Geometry check sheet. Reference: the model listing, model coordinates, mm. A direction names the side the tool comes from. Give positions to 0.01 mm unless a question says otherwise; leave off trailing zeros. Write each loop counter-clockwise with the first axis right and the second up, starting at its lowest first coordinate (ties: lowest second). Pieces come first, ordered by that corner, then holes.
(1) Cross-section at D-D (z = -24.5). Record the boundary of the cut face in (x, y), and give its area (3 significant figures).
(2) Tool access check on faces 1 (the cylindrical face through (123.767, 0.021, -65.778)), 2 (the cylindrical face through (180.594, 0.021, -25.778)). Record the directions out of +Z, -Z, +X, -X, +Y, -Y that give a thin tool (end or side, any length) a straight path to the whole face; none if there is none.
(3) Cross-section at B-B (x = -94.5). Record the boundary of the cut face in (y, z), and give its area (3 significant figures).
(4) Depth check by flat-ended pin: P1, Ø1.5, axis at y = 0, z = -4.5, coming from the +X side; P2, Ø0.9, axis at y = -0.5, z = -73, coming from the +X side; P3, Ø2.5, axis at x = -101.25, z = -43.75, coming from the -Y side; P4, Ø1.5, axis at y = 0, z = -9.5, coming from the -X side. Enter the tip coordinate at first touch or a pass-through.
(5) Cross-section at A-A (y = 0.95). Count the separate pieces of the cut face and the enclosed holes in it, and give its area (3 significant figures).
(6) Thickness scan on line 1 along X through (y, z) = (0.2, -79); line 2 along X through (y, z) = (-0.5, -65.5); line 3 along Z through (x, y) = (113.5, -0.1). Record the ranges inside material, lowest first.
(7) Mould release check, pull along X, two halves, no side actions. Record for faces 3 (the flat face through (-3, 1.5, -71)), 4 (the cylindrical face through (59.49, 0.02, 10.9)), 5 (the cylindrical face through (-121.62, 0.02, -63.68)), 6 (the cylindrical face through (121.62, 0.02, -63.68)): +X half, -X half, draft (parallel to the pull), parting line (faces both ways), or undercut.
```python
from build123d import *

# Parameters (mm, degrees)
BOSS_EXTRUDE1_DEPTH      = 1.5
BOSS_EXTRUDE1_DEPTH_BACK = 1.5
SKETCH1_W                = 125
SKETCH1_H                = 27.5
FILLET1_R                = 10
FILLET2_R                = 10
BOSS_EXTRUDE2_DEPTH      = 1.5
BOSS_EXTRUDE2_DEPTH_BACK = 1.5
SKETCH3_W                = 384
SKETCH3_H                = 110
FILLET3_R                = 40
FILLET4_R                = 40
CUT_EXTRUDE1_DEPTH       = 229.444878472
FILLET5_R                = 40
FILLET5_OF_MIRROR1_R     = 40
SKETCH5_R                = 1.5
CUT_EXTRUDE2_DEPTH       = 229.444878611
SKETCH8_W                = 3
SKETCH8_H                = 3
CUT_REVOLVE1_ANGLE       = 90


with BuildPart() as part:
    # Sketch1 → Boss-Extrude1 (new, two sides: drawn at the far end of the back side and taken through both)
    with BuildSketch(Plane(origin=(0, 0, 0), x_dir=(1, 0, 0), z_dir=(0, 1, 0)).offset(-BOSS_EXTRUDE1_DEPTH_BACK)):
        Rectangle(SKETCH1_W, SKETCH1_H)
    extrude(amount=BOSS_EXTRUDE1_DEPTH + BOSS_EXTRUDE1_DEPTH_BACK)

    # Fillet1
    fillet1_edges = [part.edges().sort_by_distance(p)[0] for p in [
        (-62.5, 0, 13.75),
    ]]
    fillet(fillet1_edges, radius=FILLET1_R)

    # Fillet2
    fillet2_edges = [part.edges().sort_by_distance(p)[0] for p in [
        (62.5, 0, 13.75),
    ]]
    fillet(fillet2_edges, radius=FILLET2_R)

    # Sketch3 → Boss-Extrude2 (add, two sides: drawn at the far end of the back side and taken through both)
    with BuildSketch(Plane(origin=(0, 0, 0), x_dir=(1, 0, 0), z_dir=(0, 1, 0)).offset(-BOSS_EXTRUDE2_DEPTH_BACK)):
        with Locations((0, 68.75)):
            Rectangle(SKETCH3_W, SKETCH3_H)
    extrude(amount=BOSS_EXTRUDE2_DEPTH + BOSS_EXTRUDE2_DEPTH_BACK)

    # Fillet3
    fillet3_edges = [part.edges().sort_by_distance(p)[0] for p in [
        (192, 0, -13.75),
    ]]
    fillet(fillet3_edges, radius=FILLET3_R)

    # Fillet4
    fillet4_edges = [part.edges().sort_by_distance(p)[0] for p in [
        (-192, 0, -13.75),
    ]]
    fillet(fillet4_edges, radius=FILLET4_R)

    # Sketch4 → Cut-Extrude1 (cut, through all)
    with BuildSketch(Plane(origin=(0, 1.5, 0), x_dir=(1, 0, 0), z_dir=(0, 1, 0))):
        with BuildLine():
            Line((-160.390648589, 123.75), (-192, 123.75))
            Line((-192, 123.75), (-192, 61.83266327))
            add(Edge.make_bspline(
                [(-192, 61.83266327), (-190.899009452, 93.759296174), (-172, 113.75)],
                knots=[0.088627388, 0.088627388, 0.088627388, 0.804978643, 0.804978643, 0.804978643], degree=2))
            add(Edge.make_bspline(
                [(-172, 113.75), (-166.85488377, 119.192321989), (-160.390648589, 123.75)],
                knots=[0.804978643, 0.804978643, 0.804978643, 1, 1, 1], degree=2))
        make_face()
        with BuildLine():
            Line((-142, 123.75), (-160.390648589, 123.75))
            add(Edge.make_bspline(
                [(-172, 113.75), (-166.85488377, 119.192321989), (-160.390648589, 123.75)],
                knots=[0.804978643, 0.804978643, 0.804978643, 1, 1, 1], degree=2))
            add(Edge.make_bspline(
                [(-172, 113.75), (-157.601214668, 122.454851717), (-142, 123.75)],
                knots=[0, 0, 0, 0.740970343, 0.740970343, 0.740970343], degree=2))
        make_face()
    cut_extrude1 = extrude(amount=-CUT_EXTRUDE1_DEPTH, mode=Mode.SUBTRACT)

    # Fillet5
    fillet5_edges = [part.edges().sort_by_distance(p)[0] for p in [
        (-172, 0, -113.75),
    ]]
    fillet(fillet5_edges, radius=FILLET5_R)

    # Mirror1: Cut-Extrude1 across plane
    add(cut_extrude1.mirror(Plane(origin=(0, 0, 0), x_dir=(0, 0, 1), z_dir=(1, 0, 0))), mode=Mode.SUBTRACT)

    # Fillet5 of Mirror1
    fillet5_of_mirror1_edges = [part.edges().sort_by_distance(p)[0] for p in [
        (172, 0, -113.75),
    ]]
    fillet(fillet5_of_mirror1_edges, radius=FILLET5_OF_MIRROR1_R)

    # Sketch5 → Cut-Extrude2 (cut, through all)
    with BuildSketch(Plane(origin=(0, 1.5, 0), x_dir=(1, 0, 0), z_dir=(0, 1, 0))):
        with Locations(Location((-101.25, 43.75, 0), (0, 0, 270))):
            Circle(SKETCH5_R)
        with Locations(Location((-131.25, 43.75, 0), (0, 0, 270))):
            Circle(SKETCH5_R)
        with Locations(Location((-161.25, 43.75, 0), (0, 0, 270))):
            Circle(SKETCH5_R)
    cut_extrude2 = extrude(amount=-CUT_EXTRUDE2_DEPTH, mode=Mode.SUBTRACT)

    # Sketch8 → Cut-Revolve1 (revolve, cut)
    with BuildSketch(Plane.XY.offset(-43.75)):
        with Locations((-131.25, 0)):
            Rectangle(SKETCH8_W, SKETCH8_H)
        with Locations((-161.25, 0)):
            Rectangle(SKETCH8_W, SKETCH8_H)
    cut_revolve1 = revolve(axis=Axis((-101.25, -1.5, -43.75), (0, -1, 0)), revolution_arc=CUT_REVOLVE1_ANGLE, mode=Mode.SUBTRACT)

    # Mirror2: Cut-Extrude2, Cut-Revolve1 across plane
    add(cut_extrude2.mirror(Plane(origin=(0, 0, 0), x_dir=(0, 0, 1), z_dir=(1, 0, 0))), mode=Mode.SUBTRACT)
    add(cut_revolve1.mirror(Plane(origin=(0, 0, 0), x_dir=(0, 0, 1), z_dir=(1, 0, 0))), mode=Mode.SUBTRACT)


solid = part.part
```
Reply:
1. outline: (-179.28, -1.5) - (179.28, -1.5) - (179.28, 1.5) - (-179.28, 1.5) - close
1. area: 1,080 mm2
2. face 1: +Y, -Y
2. face 2: +Z, +X, +Y, -Y
3. outline: (-1.5, -123.75) - (1.5, -123.75) - (1.5, -13.75) - (-1.5, -13.75) - close
3. area: 330 mm2
4. P1: stops at x = 62.5
4. P2: stops at x = 191.08
4. P3: passes through
4. P4: stops at x = -62.5
5. separate pieces: 1
5. enclosed holes: 6
5. area: 42,800 mm2
6. line 1: x = -189.94 to -151.65, -147.94 to 147.94, 151.65 to 189.94
6. line 2: x = -191.81 to -158.78, -155.56 to -124.04, -119.67 to 119.67, 124.04 to 155.56, 158.78 to 191.81
6. line 3: z = -123.75 to -104.02, -100.95 to -72.77, -69.48 to -13.75
7. face 3: draft
7. face 4: +X half
7. face 5: undercut
7. face 6: undercut
